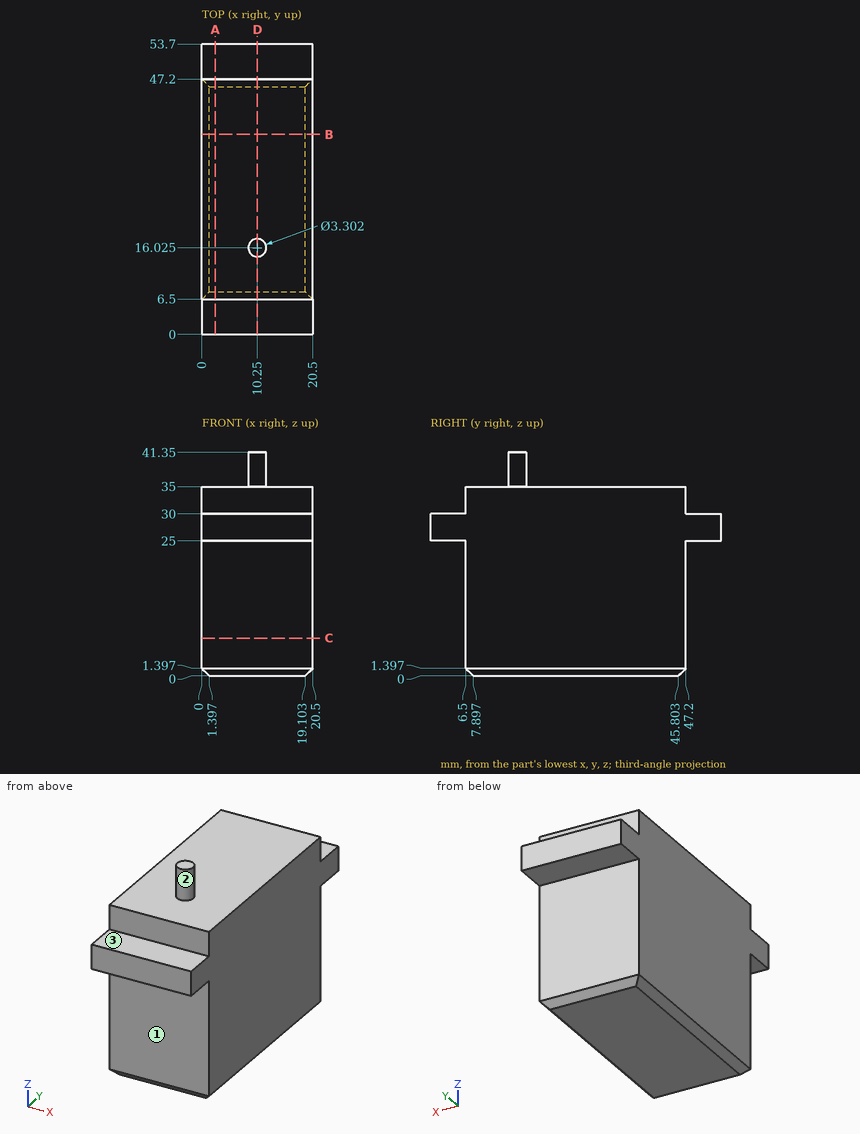
Here's the drawing with two shaded views (mm, measured from the low corner). I have some questions. A direction names the side the tool comes from. Give positions to 0.01 mm unless a question says otherwise; leave off trailing zeros. Write each loop counter-clockwise with the first axis right and the second up, starting at its lowest first coordinate (ties: lowest second). Pieces come first, ordered by that corner, then holes. Notation, with made-up numbers: (-12, 16) - (23, 16) arc R23 cw to (23, 28) - close; hole circle Ø8 at (49, 12). An arc over 180 degrees is marked (long way). One line per item, written item: value. Start each with the question number.
Item 1: Please list where these lines run through material, in increasing order: line 1 (Z direction, x = 16.5, y = 14); line 2 (Y direction, x = 15, z = 2.5); line 3 (Z direction, x = 2.5, y = 6). Write a range as from..to.
Item 2: Imagine slicing it at C-C, the plane z = 7. List the corners of the cut face in (x, y) for me.
Item 3: Which directions (+Z, -Z, +X, -X, +Y, -Y) give clear straight access to the entire face, cutting with the end or side of a thin tool? Please do the marked faces 1, 2 and 3.
Item 4: Imagine slicing it at B-B, the plane y = 37. List the corners of the cut face in (x, z) for me, and give its area (3 significant figures).
Item 5: Imagine slicing it at D-D, the plane x = 10.25. List the corners of the cut face in (y, z) for me.
Item 6: I'm going to push flat-ended pins straight in: pin 1 (5 mm diameter, centred on x = 7.5, y = 2.5, fed in from +Z); pin 2 (4 mm diameter, centred on x = 12, y = 36.5, fed in from +Z); pin 3 (2 mm diameter, centred on x = 9.5, y = 2, fed in from -Z). Where does each tip first touch, or does it pass through?
Item 7: Imagine slicing it at A-A, the plane x = 2.5. List the corners of the cut face in (y, z) for me, and give its area (3 significant figures).
Geometry says:
1. line 1: 0..35
1. line 2: 6.5..47.2
1. line 3: 25..30
2. outline: (0, 6.5) - (20.5, 6.5) - (20.5, 47.2) - (0, 47.2) - close
3. face 1: -Z, +X, -X, -Y
3. face 2: +Z
3. face 3: +Z, +X, -X, -Y
4. outline: (0, 1.4) - (1.4, 0) - (19.1, 0) - (20.5, 1.4) - (20.5, 35) - (0, 35) - close
4. area: 716 mm^2
5. outline: (0, 25) - (6.5, 25) - (6.5, 1.4) - (7.9, 0) - (45.8, 0) - (47.2, 1.4) - (47.2, 25) - (53.7, 25) - (53.7, 30) - (47.2, 30) - (47.2, 35) - (17.68, 35) - (17.68, 41.35) - (14.37, 41.35) - (14.37, 35) - (6.5, 35) - (6.5, 30) - (0, 30) - close
6. pin 1: z = 30
6. pin 2: z = 35
6. pin 3: z = 25
7. outline: (0, 25) - (6.5, 25) - (6.5, 1.4) - (7.9, 0) - (45.8, 0) - (47.2, 1.4) - (47.2, 25) - (53.7, 25) - (53.7, 30) - (47.2, 30) - (47.2, 35) - (6.5, 35) - (6.5, 30) - (0, 30) - close
7. area: 1,490 mm^2
